Autodesk Inventor part; units mm, degrees
ref_plane "YZ Plane" through (0, 0, 0) normal (1, 0, 0) x (0, 1, 0)
ref_plane "XZ Plane" through (0, 0, 0) normal (0, 1, 0) x (-1, 0, 0)
ref_plane "XY Plane" through (0, 0, 0) normal (0, 0, 1) x (1, 0, 0)
sketch "Sketch1" plane through (0, 0, 0) normal (0, 1, 0) x (-1, 0, 0)
  line L0 (0, 0) -> (0, 81.1234)
  line L1 (76.8, 81.1234) -> (80, 81.1234)
  line L2 (0, 81.1234) -> (76.8, 81.1234) construction
  line L3 (80, 81.1234) -> (83.13, 74.6607)
  line L4 (83.13, 34.4) -> (87.45, 34.4)
  line L5 (87.45, 34.4) -> (87.45, 8.8)
  line L6 (87.45, 8.8) -> (82.65, 8.8)
  line L7 (82.65, 8.8) -> (82.65, 0)
  line L8 (82.65, 0) -> (80.25, 0)
  line L9 (80.25, 0) -> (80.25, 11.2)
  line L10 (80.25, 11.2) -> (85.05, 11.2)
  line L11 (85.05, 11.2) -> (85.05, 32)
  line L12 (85.05, 32) -> (80.25, 32)
  line L13 (80.25, 32) -> (80.25, 74)
  line L14 (80.25, 74) -> (76.8, 81.1234)
  line L15 (80.25, 0) -> (0, 0) construction
  line L16 (83.13, 74.6607) -> (83.13, 34.4)
  line L17 (0, 81.1234) -> (0, 171.1234) construction
  line L18 (0, 171.1234) -> (-90, 171.1234) construction
  line L19 (-90, 171.1234) -> (-171.1234, 171.1234) construction
  line L20 (-171.1234, 171.1234) -> (-171.1234, 251.3734) construction
  line L21 (-171.1234, 251.3734) -> (-171.1234, 253.7734)
  line L22 (-171.1234, 253.7734) -> (-162.3234, 253.7734)
  line L23 (-162.3234, 253.7734) -> (-162.3234, 258.5734)
  line L24 (-162.3234, 258.5734) -> (-136.7234, 258.5734)
  line L25 (-136.7234, 258.5734) -> (-136.7234, 254.2534)
  line L26 (-136.7234, 254.2534) -> (-96.4626, 254.2534)
  line L27 (-96.4626, 254.2534) -> (-90, 251.1234)
  line L28 (-90, 251.1234) -> (-90, 247.9234)
  line L29 (-90, 247.9234) -> (-97.1234, 251.3734)
  line L30 (-97.1234, 251.3734) -> (-139.1234, 251.3734)
  line L31 (-139.1234, 251.3734) -> (-139.1234, 256.1734)
  line L32 (-139.1234, 256.1734) -> (-159.9234, 256.1734)
  line L33 (-159.9234, 256.1734) -> (-159.9234, 251.3734)
  line L34 (-159.9234, 251.3734) -> (-171.1234, 251.3734)
  line L35 (-90, 247.9234) -> (-90, 171.1234) construction
  line L36 (80.25, 74) -> (0, 74) construction
  line L37 (-97.1234, 251.3734) -> (-97.1234, 171.1234) construction
  dimension "d0" = 2.4
  dimension "d1" = 2.4
  dimension "d2" = 2.4
  dimension "d4" = 2.88
  dimension "d5" = 2.4
  dimension "d6" = 7.2
  dimension "d7" = 160.5
  dimension "d8" = 32
  dimension "d9" = 42
  dimension "d11" = 11.2
  dimension "d12" = 160
  dimension "d13" = 3.2
  dimension "d14" = 2.88
  dimension "d17" = 160.5
  dimension "d18" = 2.4
  dimension "d19" = 2.4
  dimension "d20" = 2.4
  dimension "d21" = 2.4
  dimension "d22" = 4.8
  dimension "d23" = 2.88
  dimension "d24" = 3.2
  dimension "d25" = 160
  dimension "d26" = 11.2
  dimension "d27" = 32
  dimension "d28" = 42
  dimension "d29" = 90
  dimension "d30" = 90
  dimension "d31" = 2.88
revolve "Revolution1" add sketch "Sketch1" angle 360 about axis through (0, 0, 0) along (0, 0, 1) contours L1 L3 L16 L4 L5 L6 L7 L8 L9 L10 L11 L12 L13 L14
sketch "Sketch2" plane through (0, 0, 81.1234) normal (0, 0, 1) x (1, 0, 0)
  circle A0 centre (0, 0) radius 80
  circle A1 centre (0, 0) radius 80
  circle A2 centre (0, 0) radius 76.8
  circle A3 centre (0, 0) radius 76.8
sketch "Sketch3" plane through (0, 0, 0) normal (0, 1, 0) x (-1, 0, 0)
  line L0 (-80, 81.1234) -> (80, 81.1234)
  line L1 (0, 81.1234) -> (0, 171.1234) construction
  line L2 (0, 171.1234) -> (-90, 171.1234) construction
  arc A0 (0, 81.1234) -> (-90, 171.1234) centre (-90, 81.1234) ccw
  dimension "d15" = 90
  dimension "d16" = 90
sweep "Sweep1" add profiles "Sketch2" path "Sketch3" path curves A0
revolve "Revolution2" add sketch "Sketch1" angle 360 about axis through (90, 0, 171.1234) along (1, 0, 0) contours L21 L22 L23 L24 L25 L26 L27 L28 L29 L30 L31 L32 L33 L34
equation "\"d0\" = e3"
equation "\"d1\" = e3"
equation "\"d2\" = e3"
equation "\"d4\" = e2"
equation "\"d5\" = e3"
equation "\"d6\" = 3 * e3"
equation "\"d7\" = Ds"
equation "\"d8\" = C1"
equation "\"d9\" = A"
equation "\"d11\" = 0.35 * C1"
equation "\"d12\" = De"
equation "\"d13\" = e"
equation "\"d14\" = e2"
equation "\"d17\" = Ds"
equation "\"d18\" = e3"
equation "\"d19\" = e3"
equation "\"d20\" = e3"
equation "\"d21\" = e3"
equation "\"d22\" = 2 * e3"
equation "\"d23\" = e2"
equation "\"d24\" = e"
equation "\"d25\" = De"
equation "\"d26\" = 0.35 * C1"
equation "\"d27\" = C1"
equation "\"d28\" = A"
equation "\"d29\" = z"
equation "\"d30\" = z"
equation "\"d31\" = e2"
equation "\"d15\" = z"
equation "\"d16\" = z"
equation "\"z\" = 90"
equation "\"De\" = 160"
equation "\"e\" = 3.2"
equation "\"Ds\" = 160.5"
equation "\"e2\" = 0.9 * e"
equation "\"C1\" = 32"
equation "\"e3\" = 0.75 * e"
equation "\"A\" = 42"
equation "\"Size_Designation\" = 1.2345"
properties part number "ISO 3633 90 Deg Bend with Only Sockets for Elastormeric Sealing Ring Joints DN160" material "PVC, Unplasticized"
Part model, mm, in its own coordinate system. A direction names the side the tool comes from. Give positions to 0.01 mm unless a question says otherwise; leave off trailing zeros. Loops run counter-clockwise (first coordinate to the right, second up) from the corner with the lowest first, then second, coordinate; pieces in that order, holes last. Notation, with made-up numbers: (46.5, 85) -> (105.5, 85) arc R23 ccw to (105.5, 104) -> close; hole circle Ø11 at (43.25, 74.5). An arc over 180 degrees is marked (long way). Write each question's results on one line, items separated by ' | '. Start each with the question number.
Q1. Band-saw the part on A-A on x = 125.5. List the corners of the cut face in (y, z), plus the area to 3 significant figures.
Q2. Pin check, flat tips, straight feed: P1, Ø8, axis at x = 131, z = 132, coming from the -Y side; P2, Ø1.5, axis at x = 128.5, y = 46, coming from the -Z side; P3, Ø8, axis at y = -2, z = 171, coming from the -X side. Stop position of each tip, or through.
Q3. Pull direction Y, two halves, no side cores. Call faces 5 (the face through (149.669, -25.547, 252.246)), 6 (the face through (90.404, -24.089, 247.616)), 7 (the face through (162.323, -52.2, 235.5)): +Y half, -Y half, draft (parallel to the pull), parting line (faces both ways), or undercut.
Q4. Which spindle directions (+Z, -Z, +X, -X, +Y, -Y) get a long thin tool onto all of the face, cutting with end or side? Do faces 1 (the face through (68, -43, 0)), 2 (the face through (149.34, 3.85, 83.76)), 3 (the face through (51, 63, 32)), 4 (the face through (18.96, -85.37, 21.42)). Say none if no direction does.
Q5. Wall check: L1, parallel to Y at x = 0, z = 58; L2, parallel to Y at x = 0, z = 21.5; L3, parallel to Z at x = 149.5, y = 0. Give the ranges that are in metal, low to high.
Q6. Band-saw the part on B-B on z = 41. List the corners of the cut face in (x, y), plus the area to 3 significant figures.
Results are:
1) outline: circle Ø166.26 at (0, 171.12); hole circle Ø160.5 at (0, 171.12) | area: 1,480 mm²
2) P1: stops at y = -75.35 | P2: stops at z = 101.39 | P3: stops at x = -56.69
3) face 5: undercut | face 6: parting line | face 7: draft
4) face 1: -Z, +X, -X, +Y, -Y | face 2: +X | face 3: none | face 4: -Z
5) L1: y = -83.13 to -80.25, 80.25 to 83.13 | L2: y = -87.45 to -85.05, 85.05 to 87.45 | L3: z = 83.67 to 86.07, 256.17 to 258.57
6) outline: circle Ø166.26 at (0, 0); hole circle Ø160.5 at (0, 0) | area: 1,480 mm²
